from build123d import *

# Parameters (mm, degrees)
SKETCH_1_W                         = 200
SKETCH_1_H                         = 40
EXTRUDE_1_DEPTH                    = 13
SWEEP_START                        = -100
SWEEP_1_DEPTH                      = 200
SWEEP_2_DEPTH                      = 200
SKETCH_16_R                        = 4.075
CUT_EXTRUDE_1_DEPTH                = 2.15
PATTERN_LINEAR_1_COUNT             = 2
PATTERN_LINEAR_1_PITCH             = 80
PATTERN_CIRCULAR_1_COUNT           = 2
PATTERN_CIRCULAR_1_COPY_1_SKETCH_R = 4.075
PATTERN_CIRCULAR_1_COPY_1_DEPTH    = 2.15
SKETCH_20_R                        = 4.075
CUT_EXTRUDE_2_DEPTH                = 2.15
FILLET_1_R                         = 5


# Read off the part's stored shape, not the designer's step: Вырез-По траектории1, Вырез-По траектории2
with BuildPart() as part:
    # Эскиз1 → Бобышка-Вытянуть1 (new body)
    with BuildSketch(Plane(origin=(0, 0, 0), x_dir=(1, 0, 0), z_dir=(0, 1, 0))):
        Rectangle(SKETCH_1_W, SKETCH_1_H)
    extrude(amount=-EXTRUDE_1_DEPTH)

    # Вырез-По траектории1 outline → Вырез-По траектории1 (cut)
    with BuildSketch(Plane.YZ.offset(SWEEP_START)):
        with BuildLine():
            Line((0, 20), (-1.5, 20))
            ThreePointArc((-1.5, 20), (-1.060660172, 18.939339828), (0, 18.5))
            Line((0, 18.5), (0, 20))
        make_face()
    extrude(amount=SWEEP_1_DEPTH, mode=Mode.SUBTRACT)

    # Вырез-По траектории2 outline → Вырез-По траектории2 (cut)
    with BuildSketch(Plane.YZ.offset(SWEEP_START)):
        with BuildLine():
            ThreePointArc((0, -18.5), (-1.060660172, -18.939339828), (-1.5, -20))
            Line((-1.5, -20), (0, -20))
            Line((0, -20), (0, -18.5))
        make_face()
    extrude(amount=SWEEP_2_DEPTH, mode=Mode.SUBTRACT)

    # Эскиз16 → Вырез-Вытянуть1 (cut)
    with BuildSketch(Plane(origin=(0, 0, -20), x_dir=(-1, 0, 0), z_dir=(0, 0, -1))):
        with Locations((-60, -7.565202347)):
            Circle(SKETCH_16_R)
        with BuildLine():
            Line((-60, -2.859797653), (-62.0375, -4.036148827))
            ThreePointArc((-62.0375, -4.036148827), (-60, -3.490202347), (-57.9625, -4.036148827))
            Line((-57.9625, -4.036148827), (-60, -2.859797653))
        make_face()
    cut_extrude_1 = extrude(amount=-CUT_EXTRUDE_1_DEPTH, mode=Mode.SUBTRACT)

    # Линейный массив1: Вырез-Вытянуть1 ×2
    with Locations(*[(-i * PATTERN_LINEAR_1_PITCH, 0, 0) for i in range(1, PATTERN_LINEAR_1_COUNT)]):
        add(cut_extrude_1, mode=Mode.SUBTRACT)

    # Круговой массив1: Вырез-Вытянуть1 ×2 about axis
    pattern_circular_1_axis = Axis((0, -13, 0), (0, -1, 0))
    for i in range(1, PATTERN_CIRCULAR_1_COUNT):
        add(cut_extrude_1.rotate(pattern_circular_1_axis, i * 360 / PATTERN_CIRCULAR_1_COUNT), mode=Mode.SUBTRACT)

    # Круговой массив1 copy 1 sketch → Круговой массив1 copy 1 (cut)
    with BuildSketch(Plane(origin=(80, 0, 20), x_dir=(1, 0, 0), z_dir=(0, 0, 1))):
        with Locations((-60, -7.565202347)):
            Circle(PATTERN_CIRCULAR_1_COPY_1_SKETCH_R)
        with BuildLine():
            Line((-60, -2.859797653), (-62.0375, -4.036148827))
            ThreePointArc((-62.0375, -4.036148827), (-60, -3.490202347), (-57.9625, -4.036148827))
            Line((-57.9625, -4.036148827), (-60, -2.859797653))
        make_face()
    extrude(amount=-PATTERN_CIRCULAR_1_COPY_1_DEPTH, mode=Mode.SUBTRACT)

    # Эскиз20 → Вырез-Вытянуть2 (cut)
    with BuildSketch(Plane.ZY.offset(-100)):
        with Locations((0, -6.815202347)):
            Circle(SKETCH_20_R)
        with BuildLine():
            Line((2.0375, -3.286148827), (0, -2.109797653))
            Line((0, -2.109797653), (-2.0375, -3.286148827))
            ThreePointArc((-2.0375, -3.286148827), (0, -2.740202347), (2.0375, -3.286148827))
        make_face()
    extrude(amount=CUT_EXTRUDE_2_DEPTH, mode=Mode.SUBTRACT)

    # Скругление1
    fillet_1_edges = [part.edges().sort_by_distance(p)[0] for p in [
        (-100, 0, 0),
    ]]
    fillet(fillet_1_edges, radius=FILLET_1_R)


solid = part.part
Design review of the part built by this model. Coordinates are the model's own, in mm. A direction names the side the tool comes from. Round coordinates to 2 decimals unless told otherwise and drop trailing zeros.
Item 1: Draft analysis for pull direction X (two halves, no side actions). For faces 1 (the cylindrical face through (19.851, -11.637, 18.94)), 2 (the flat face through (97.85, -6, 0)), 3 (the flat face through (-100, -9, 0)), state which applies: released by +X, released by -X, zero draft, split by the parting line, or undercut.
Item 2: Wall thickness on L1, parallel to Y at x = -60, z = 18; L2, parallel to X at y = -4.25, z = -18; L3, parallel to Y at x = 20, z = 19.1: over which ranges is each line inside the solid? List them lowest first.
Item 3: For pin 1 Ø6.5 at (x, y) = (-20, -7.57) entering from -Z; pin 2 Ø6.5 at (x, y) = (-60, -6.5) entering from +Z; pin 3 Ø5 at (x, y) = (-60, -7.57) entering from +Z, all flat-tipped, find the tip position at first contact; note any pin that passes through.
Item 4: For faces 4 (the flat face through (-1, -7, 20)), 5 (the cylindrical face through (-60.149, -11.637, 18.94)), 6 (the cylindrical face through (98.94, -10.887, -0.149)), 7 (the flat face through (-1, -7, -20)), 8 (the cylindrical face through (-19.851, -11.637, -18.94)), list the 3-axis set-ups (+Z, -Z, +X, -X, +Y, -Y) from which the entire face can be reached by the end or side of a thin tool; tool diameter is ignored.
Check values:
1. face 1: undercut
1. face 2: released by +X
1. face 3: released by -X
2. L1: y = -13 to -11.64, -2.86 to 0
2. L2: x = -99.94 to -22.37, -17.63 to 57.63, 62.37 to 100
2. L3: y = -13 to -11.64, -2.86 to -1.2
3. pin 1: stops at z = -17.85
3. pin 2: stops at z = 20
3. pin 3: stops at z = 17.85
4. face 4: +Z, +X, -X, +Y, -Y
4. face 5: +Z
4. face 6: +X
4. face 7: -Z, +X, -X, +Y, -Y
4. face 8: -Z
